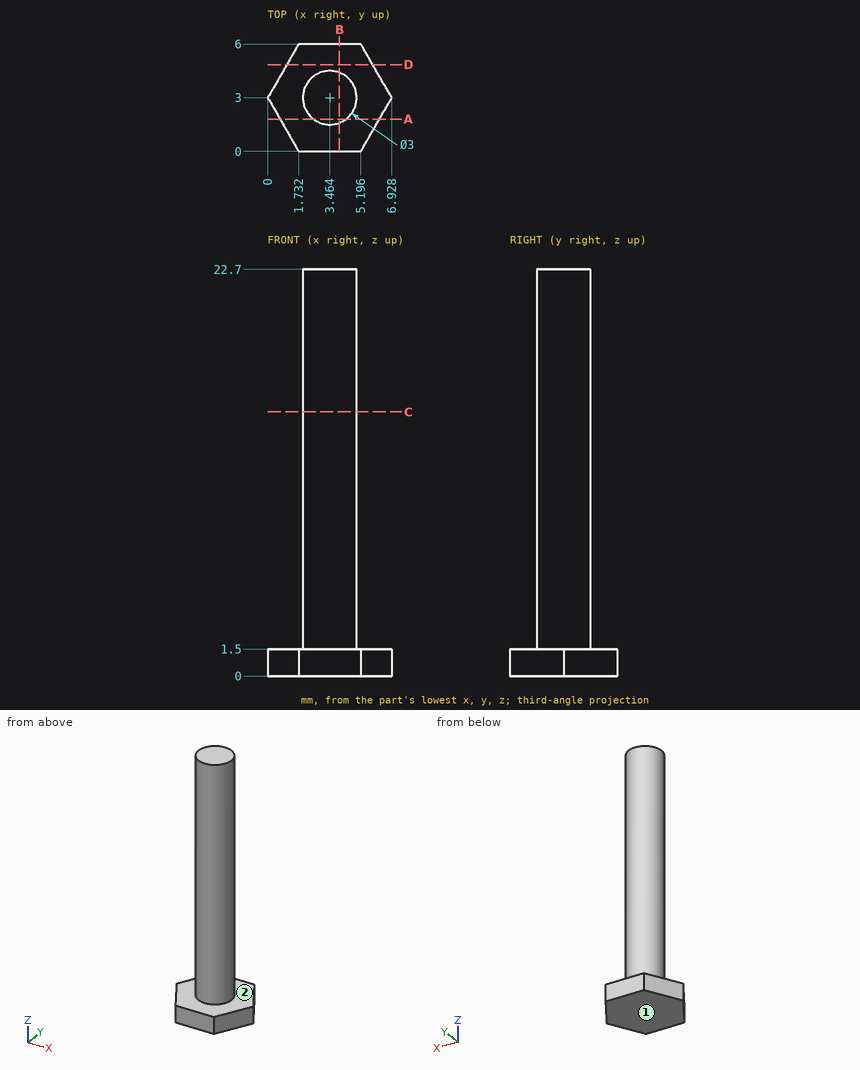
Job drawing, mm, ordinate dimensions from the low corner. One solid piece. A direction names the side the tool comes from. Give positions to 0.01 mm unless a question says otherwise; leave off trailing zeros. Write each loop counter-clockwise with the first axis right and the second up, starting at its lowest first coordinate (ties: lowest second). Pieces come first, ordered by that corner, then holes. Notation, with made-up numbers: (68.5, 61) - (87.5, 61) arc R5 ccw to (87.5, 70) - close; hole circle Ø4 at (9, 44). An arc over 180 degrees is marked (long way). Use one line per item in the form item = value. Start each with the question number.
1. Band-saw the part on D-D on y = 4.85. Write the cut outline in (x, z).
2. Drop flat-ended pins along their axis: pin 1 Ø3 at (y, z) = (0.5, 13.5) entering from +X; pin 2 Ø2 at (y, z) = (4, 3.5) entering from +X; pin 3 Ø1.5 at (y, z) = (4, 11.5) entering from +X; pin 4 Ø3 at (x, y) = (5.5, 2) entering from -Z. Give the stop position or say it passes through.
3. Band-saw the part on A-A on y = 1.8. Write the cut outline in (x, z) (1 decimal), plus the area to 3 significant figures.
4. 3-axis set-ups, long thin cutter, end or side, ignore diameter. For the marked faces 1 and 2: which of +Z, -Z, +X, -X, +Y, -Y reach the whole face in a straight line?
5. Band-saw the part on B-B on x = 4. Write the cut outline in (y, z).
6. Probe line 1 (Z direction, x = 2, y = 1.7); line 2 (X direction, y = 1.95, z = 5.5) (1 decimal); line 3 (X direction, y = 2.3, z = 18.25). List the from-to ranges inside material, lowest first. Write a range as [from, to].
7. Band-saw the part on C-C on z = 14.75. Write the cut outline in (x, y).
Conclusion:
q1.outline = (1.07, 0) - (5.86, 0) - (5.86, 1.5) - (1.07, 1.5) - close
q2.pin_1 = 4.58
q2.pin_2 = 4.96
q2.pin_3 = 4.94
q2.pin_4 = 0
q3.outline = (0.7, 0) - (6.2, 0) - (6.2, 1.5) - (4.4, 1.5) - (4.4, 22.7) - (2.6, 22.7) - (2.6, 1.5) - (0.7, 1.5) - close
q3.area = 46.5 mm²
q4.face_1 = -Z, +X, -X, +Y, -Y
q4.face_2 = +Z
q5.outline = (0, 0) - (6, 0) - (6, 1.5) - (4.4, 1.5) - (4.4, 22.7) - (1.6, 22.7) - (1.6, 1.5) - (0, 1.5) - close
q6.line_1 = [0, 1.5]
q6.line_2 = [2.4, 4.5]
q6.line_3 = [2.14, 4.79]
q7.outline = circle Ø3 at (3.46, 3)
